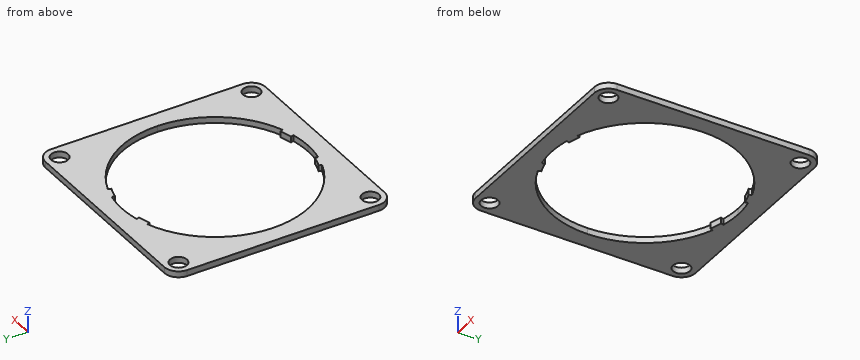
```python
from build123d import *

# Parameters (mm, degrees)
SKETCH004_R                = 4.2
PAD001_DEPTH               = 3
SKETCH004_MIRRORED003_2_R  = 4.2
PAD001_MIRRORED003_2_DEPTH = 3


with BuildPart() as part:
    # Sketch004 → Pad001 (new body)
    with BuildSketch(Plane.XY):
        with BuildLine():
            ThreePointArc((46.15, 0), (37.838009, 26.421725), (15.896152, 43.325914))
            Line((15.379484, 41.917705), (15.896152, 43.325914))
            ThreePointArc((15.379484, 41.917705), (12.528311, 42.856317), (9.620516, 43.60124))
            Line((9.620516, 43.60124), (9.943714, 45.066008))
            ThreePointArc((9.943714, 45.066008), (5.001312, 45.878202), (0, 46.15))
            Line((0, 46.15), (0, 54.625))
            Line((47.624993, 54.625), (0, 54.625))
            ThreePointArc((54.625, 47.625), (52.574745, 52.57475), (47.624993, 54.625))
            Line((54.625, 47.625), (54.625, 0))
            Line((46.15, 0), (54.625, 0))
        make_face()
        with Locations((47.625, 47.625)):
            Circle(SKETCH004_R, mode=Mode.SUBTRACT)
    pad001 = extrude(amount=PAD001_DEPTH)

    # Sketch004 Mirrored003 2 → Pad001 Mirrored003 2 (add)
    with BuildSketch(Plane(origin=(0, 0, 0), x_dir=(-1, 0, 0), z_dir=(0, 0, -1))):
        with BuildLine():
            ThreePointArc((46.15, 0), (37.838009, 26.421725), (15.896152, 43.325914))
            Line((15.379484, 41.917705), (15.896152, 43.325914))
            ThreePointArc((15.379484, 41.917705), (12.528311, 42.856317), (9.620516, 43.60124))
            Line((9.620516, 43.60124), (9.943714, 45.066008))
            ThreePointArc((9.943714, 45.066008), (5.001312, 45.878202), (0, 46.15))
            Line((0, 46.15), (0, 54.625))
            Line((47.624993, 54.625), (0, 54.625))
            ThreePointArc((54.625, 47.625), (52.574745, 52.57475), (47.624993, 54.625))
            Line((54.625, 47.625), (54.625, 0))
            Line((46.15, 0), (54.625, 0))
        make_face()
        with Locations((47.625, 47.625)):
            Circle(SKETCH004_MIRRORED003_2_R, mode=Mode.SUBTRACT)
    pad001_mirrored003_2 = extrude(amount=-PAD001_MIRRORED003_2_DEPTH)

    # Mirrored004: Pad001, Pad001 Mirrored003 2 across Sketch004 H_Axis
    add(pad001.mirror(Plane.ZX))
    add(pad001_mirrored003_2.mirror(Plane.ZX))


solid = part.part
```
Work out the finished part from the listing and answer in its coordinate system (mm). Round coordinates to 2 decimals unless told otherwise and drop trailing zeros. Loops run counter-clockwise (first coordinate to the right, second up) from the corner with the lowest first, then second, coordinate; pieces in that order, holes last.
(1) The part is cut by section C-C, the plane y = 13. Give the vertices of the cut face in (x, z) (3 decimals).
Computed values:
outline: (-54.625, 0) - (-44.281, 0) - (-44.281, 3) - (-54.625, 3) - close; (44.281, 0) - (54.625, 0) - (54.625, 3) - (44.281, 3) - close
(2) Find the intervals of material crossed by L1, parallel to Y at x = -48, z = 2.75; L2, parallel to X at y = 34, z = 1.4 (3 decimals), in increasing order.
Computed values:
L1: y = -54.61 to -51.81, -43.44 to 43.44, 51.81 to 54.61
L2: x = -54.625 to -31.206, 31.206 to 54.625
(3) The part is cut by section B-B, the plane x = -28.5. Give the vertices of the cut face in (y, z) (3 decimals).
Computed values:
outline: (-54.625, 0) - (-36.298, 0) - (-36.298, 3) - (-54.625, 3) - close; (36.298, 0) - (54.625, 0) - (54.625, 3) - (36.298, 3) - close
(4) The part is cut by section A-A, the plane z = 1.7. Give the number of separate pieces and of enclosed holes in the cut face, and give its area (3 significant figures).
Computed values:
separate pieces: 1
enclosed holes: 5
area: 5,020 mm2
(5) This flat-tipped pin is pushed along its axis until it touches: P1, Ø10, axis at x = 23.5, y = -31, coming from the +Z side. Where does it stop, or does it pass through?
Computed values:
P1: passes through
